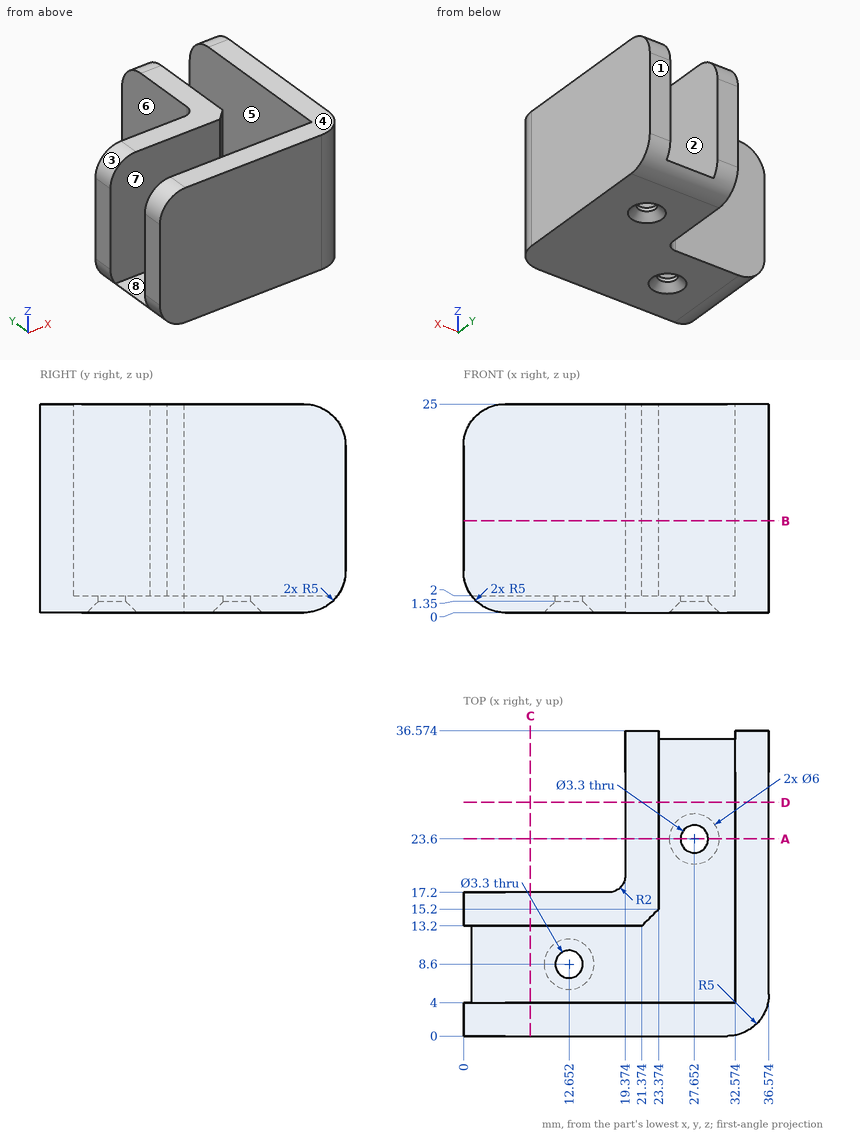
Verification items for this drawing (mm, ordinates from the low corner). A direction names the side the tool comes from. Coordinates: 2 decimals unless noted, no trailing zeros. Order: outer loops, then holes, each group sorted by start corner. A loop starts at its lowest first (then second) coordinate and runs counter-clockwise, first axis right, second up. Notation, with made-up numbers: (47, -17) - (60, -17) arc R31 cw to (60, 22) - close; hole circle Ø6 at (21, 4). An arc over 180 degrees is marked (long way). Use one line per item in the form item = value.
1. Section check C-C (x = 8). Record the boundary of the cut face in (y, z).
Here are the results:
outline = (0, 0) - (17.2, 0) - (17.2, 25) - (13.2, 25) - (13.2, 2) - (4, 2) - (4, 25) - (0, 25) - close
2. Scan lines: line 1 (X direction, y = 24, z = 19); line 2 (Y direction, x = 6.5, z = 16); line 3 (X direction, y = 23.6, z = 1.8). Record each from-to range of solid material in increasing order.
Here are the results:
line_1 = 19.37 to 23.37, 32.57 to 36.57
line_2 = 0 to 4, 13.2 to 17.2
line_3 = 19.37 to 26, 29.3 to 36.57
3. Gauge pin test, flat ends, axial feed: pin 1 (8.5 mm diameter, centred on x = 7, z = 9.5, fed in from +Y); pin 2 (5.5 mm diameter, centred on x = 27.65, y = 23.6, fed in from +Z); pin 3 (4 mm diameter, centred on y = 9.5, z = 16, fed in from -X); pin 4 (6 mm diameter, centred on y = 10.5, z = 11.5, fed in from -X). Record the tip position at first contact, or that the pin passes through.
Here are the results:
pin_1 = 17.2
pin_2 = 2
pin_3 = 32.57
pin_4 = 0
4. Section check D-D (y = 28). Record the boundary of the cut face in (x, z).
Here are the results:
outline = (19.37, 0) - (36.57, 0) - (36.57, 25) - (32.57, 25) - (32.57, 2) - (23.37, 2) - (23.37, 25) - (19.37, 25) - close
5. Draft check along X on the marked faces 1, 2 and 3. Enter one of: pulls with the +X half, pulls with the -X half, needs draft (parallel to the pull), parting line crosses it, or undercut.
Here are the results:
face_1 = needs draft
face_2 = undercut
face_3 = pulls with the -X half
6. Access from +Z, -Z, +X, -X, +Y, -Y to the whole of each face (thin tool, end or side, straight path). Record for the marked faces 4, 5, 6, 7 and 8.
Here are the results:
face_4 = +Z, +X, -X, +Y, -Y
face_5 = +Z, +Y
face_6 = +Z, -Z, -X, +Y
face_7 = +Z, -X
face_8 = +Z
7. Section check A-A (y = 23.6). Record the boundary of the cut face in (x, z), then the cut area to 3 significant figures.
Here are the results:
outline = (19.37, 0) - (24.65, 0) - (26, 1.35) - (26, 2) - (23.37, 2) - (23.37, 25) - (19.37, 25) - close; (29.3, 1.35) - (30.65, 0) - (36.57, 0) - (36.57, 25) - (32.57, 25) - (32.57, 2) - (29.3, 2) - close
area = 210 mm²
8. Section check B-B (z = 11). Record the boundary of the cut face in (x, y).
Here are the results:
outline = (0, 0) - (31.57, 0) arc R5 ccw to (36.57, 5) - (36.57, 36.57) - (32.57, 36.57) - (32.57, 4) - (0, 4) - close; (0, 13.2) - (21.37, 13.2) - (23.37, 15.2) - (23.37, 36.57) - (19.37, 36.57) - (19.37, 19.2) arc R2 cw to (17.37, 17.2) - (0, 17.2) - close
